The listing builds one solid part. Answer for the finished solid, in the listing's coordinates (mm). Face numbers are marked on the shaded views. Round coordinates to 2 decimals unless told otherwise and drop trailing zeros. Loops run counter-clockwise (first coordinate to the right, second up) from the corner with the lowest first, then second, coordinate; pieces in that order, holes last. Notation, with made-up numbers: (44.25, 1) - (69.25, 1) arc R19 ccw to (69.25, 5) - close; hole circle Ø2 at (44, 51). An arc over 180 degrees is marked (long way). One line per item, written item: value.
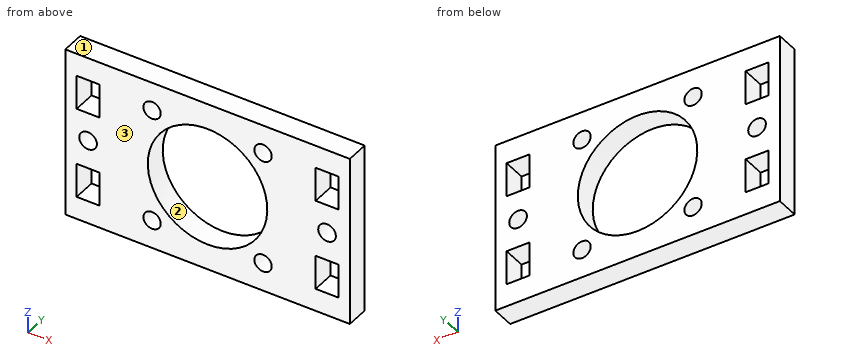
```python
from build123d import *

# Parameters (mm, degrees)
CROQUIS1_W              = 50
CROQUIS1_H              = 30
SALIENTE_EXTRUIR1_DEPTH = 4
CROQUIS2_W              = 4
CROQUIS2_H              = 6
CORTAR_EXTRUIR1_DEPTH   = 30.427877939
CROQUIS3_R              = 1.55
CORTAR_EXTRUIR2_DEPTH   = 30.427877939
CROQUIS4_R              = 10.5
CROQUIS4_R_2            = 1.525
CORTAR_EXTRUIR3_DEPTH   = 30.427877939


with BuildPart() as part:
    # Croquis1 → Saliente-Extruir1 (new body)
    with BuildSketch(Plane(origin=(0, 0, 0), x_dir=(1, 0, 0), z_dir=(0, 1, 0))):
        Rectangle(CROQUIS1_W, CROQUIS1_H)
    extrude(amount=SALIENTE_EXTRUIR1_DEPTH)

    # Croquis2 → Cortar-Extruir1 (cut, through all)
    with BuildSketch(Plane(origin=(0, 4, 0), x_dir=(1, 0, 0), z_dir=(0, 1, 0))):
        with Locations((-21, 8)):
            Rectangle(CROQUIS2_W, CROQUIS2_H)
        with Locations((-21, -8)):
            Rectangle(CROQUIS2_W, CROQUIS2_H)
        with Locations((21, -8)):
            Rectangle(CROQUIS2_W, CROQUIS2_H)
        with Locations((21, 8)):
            Rectangle(CROQUIS2_W, CROQUIS2_H)
    extrude(amount=-CORTAR_EXTRUIR1_DEPTH, mode=Mode.SUBTRACT)

    # Croquis3 → Cortar-Extruir2 (cut, through all)
    with BuildSketch(Plane(origin=(0, 4, 0), x_dir=(1, 0, 0), z_dir=(0, 1, 0))):
        with Locations(Location((-21, 0, 0), (0, 0, 270))):
            Circle(CROQUIS3_R)
        with Locations(Location((21, 0, 0), (0, 0, 90))):
            Circle(CROQUIS3_R)
    extrude(amount=-CORTAR_EXTRUIR2_DEPTH, mode=Mode.SUBTRACT)

    # Croquis4 → Cortar-Extruir3 (cut, through all)
    with BuildSketch(Plane.XZ):
        with Locations(Location((0, 0, 0), (0, 0, 270))):
            Circle(CROQUIS4_R)
        with Locations(Location((-9.75, 10, 0), (0, 0, 270))):
            Circle(CROQUIS4_R_2)
        with Locations(Location((-9.75, -10, 0), (0, 0, 270))):
            Circle(CROQUIS4_R_2)
        with Locations(Location((9.75, -10, 0), (0, 0, 270))):
            Circle(CROQUIS4_R_2)
        with Locations(Location((9.75, 10, 0), (0, 0, 270))):
            Circle(CROQUIS4_R_2)
    extrude(amount=-CORTAR_EXTRUIR3_DEPTH, mode=Mode.SUBTRACT)


solid = part.part
```
1) A cutting plane is placed at B-B on y = 1. Give the number of separate pieces and of enclosed holes in the cut face, and give its area (3 significant figures).
Final values:
separate pieces: 1
enclosed holes: 11
area: 1,010 mm2
2) Consider L1, parallel to X at y = 1, z = 0; L2, parallel to Z at x = 21, y = 2.35; L3, parallel to X at y = 1.45, z = -7.75. Determine where each line is inside the solid, lowest interval first.
Final values:
L1: -25 to -22.55, -19.45 to -10.5, 10.5 to 19.45, 22.55 to 25
L2: -15 to -11, -5 to -1.55, 1.55 to 5, 11 to 15
L3: -25 to -23, -19 to -7.08, 7.08 to 19, 23 to 25
3) A cutting plane is placed at D-D on x = 0. Give the vertices of the cut face in (y, z), and give its area (3 significant figures).
Final values:
outline: (0, -15) - (4, -15) - (4, -10.5) - (0, -10.5) - close; (0, 10.5) - (4, 10.5) - (4, 15) - (0, 15) - close
area: 36.0 mm2
4) A cutting plane is placed at A-A on x = -21. Give the vertices of the cut face in (y, z), and give its area (3 significant figures).
Final values:
outline: (0, -15) - (4, -15) - (4, -11) - (0, -11) - close; (0, -5) - (4, -5) - (4, -1.55) - (0, -1.55) - close; (0, 1.55) - (4, 1.55) - (4, 5) - (0, 5) - close; (0, 11) - (4, 11) - (4, 15) - (0, 15) - close
area: 59.6 mm2
5) For a pull along Z with two mould halves and no side action, classify the marked faces 1, 2 and 3 as released by +Z, released by -Z, zero draft, split by the parting line, or undercut.
Final values:
face 1: released by +Z
face 2: undercut
face 3: zero draft
6) A cutting plane is placed at C-C on z = 0. Give the vertices of the cut face in (x, y).
Final values:
outline: (-25, 0) - (-22.55, 0) - (-22.55, 4) - (-25, 4) - close; (-19.45, 0) - (-10.5, 0) - (-10.5, 4) - (-19.45, 4) - close; (10.5, 0) - (19.45, 0) - (19.45, 4) - (10.5, 4) - close; (22.55, 0) - (25, 0) - (25, 4) - (22.55, 4) - close
